Read the model definition and answer for the solid it produces. Units are mm, in the model's axes. A direction names the side the tool comes from. Give positions to 0.01 mm unless a question says otherwise; leave off trailing zeros. Loops run counter-clockwise (first coordinate to the right, second up) from the corner with the lowest first, then second, coordinate; pieces in that order, holes last.
(1) Find section C-C, the plane y = -9. Write down the section's boundary in (x, z), then the cut area to 3 significant figures.
(2) Each of these flat-tipped pins is pushed along its axis until it touches: P1, Ø6, axis at y = -26, z = 9, coming from the +X side; P2, Ø5, axis at x = 20.5, z = 4.5, coming from the -Y side. Where does it stop, or does it pass through?
(3) Find section B-B, the plane x = 18.25. Write down the section's boundary in (y, z), then the cut area to 3 significant figures.
(4) Find section D-D, the plane x = 0. Write down the section's boundary in (y, z).
(5) Find section A-A, the plane y = -31. Write down the section's boundary in (x, z), then the cut area to 3 significant figures.
(6) Determine the mould class of faces 4 (the face through (-0.521, -27.034, 5.07)), 5 (the face through (0, 40.074, 5)), 6 (the face through (-13.861, -31, 5)) for opening direction Y: pulls with the +Y half, pulls with the -Y half, needs draft (parallel to the pull), parting line crosses it, or undercut.
(7) Which of the six approach directions +Z, -Z, +X, -X, +Y, -Y give full straight-line access (tool end or side, diameter ignored) to faces 1 (the face through (0, 1, 0)), 2 (the face through (25, -21.926, 5)), 3 (the face through (-24, -21.926, 5))?
(8) Straight lines are drawn through the part: probe 1 along Y at (x, z) = (0, 5.5); probe 2 along Y at (x, z) = (-18, 7); probe 3 along X at (y, z) = (-9.5, 2). For each, find the intervals that lie inside material, in ascending order.
```python
from build123d import *

# Parameters (mm, degrees)
BOSS_EXTRUDE1_DEPTH = 10
SKETCH2_R           = 4
SKETCH2_R_2         = 2.5
CUT_EXTRUDE1_DEPTH  = 11
SKETCH8_R           = 12.955
CUT_EXTRUDE9_DEPTH  = 10


with BuildPart() as part:
    # Sketch1 → Boss-Extrude1 (new body)
    with BuildSketch(Plane.XY):
        Polygon((-35, 40.07390675), (35, 40.07390675), (35, -21.92609325), (13.861088822, -21.92609325), (13.861088822, -40.07390675), (-13.861088822, -40.07390675), (-13.861088822, -21.92609325), (-35, -21.92609325), align=None)
    extrude(amount=BOSS_EXTRUDE1_DEPTH)

    # Sketch2 → Cut-Extrude1 (cut, through all)
    with BuildSketch(Plane.XY.offset(10)):
        with Locations((0, -31)):
            Circle(SKETCH2_R)
        with Locations((0, -9)):
            Circle(SKETCH2_R)
        with Locations((-18.25, -9)):
            Circle(SKETCH2_R_2)
        with Locations((18.25, -9)):
            Circle(SKETCH2_R_2)
    extrude(amount=-CUT_EXTRUDE1_DEPTH, mode=Mode.SUBTRACT)

    # Sketch8 → Cut-Extrude9 (cut)
    with BuildSketch(Plane.XY.offset(10)):
        with Locations((0, 21.51390675)):
            Circle(SKETCH8_R)
    extrude(amount=-CUT_EXTRUDE9_DEPTH, mode=Mode.SUBTRACT)


solid = part.part
```
Entries:
1. outline: (-35, 0) - (-20.75, 0) - (-20.75, 10) - (-35, 10) - close; (-15.75, 0) - (-4, 0) - (-4, 10) - (-15.75, 10) - close; (4, 0) - (15.75, 0) - (15.75, 10) - (4, 10) - close; (20.75, 0) - (35, 0) - (35, 10) - (20.75, 10) - close
1. area: 520 mm2
2. P1: stops at x = 13.86
2. P2: stops at y = -21.93
3. outline: (-21.93, 0) - (-11.5, 0) - (-11.5, 10) - (-21.93, 10) - close; (-6.5, 0) - (40.07, 0) - (40.07, 10) - (-6.5, 10) - close
3. area: 570 mm2
4. outline: (-40.07, 0) - (-35, 0) - (-35, 10) - (-40.07, 10) - close; (-27, 0) - (-13, 0) - (-13, 10) - (-27, 10) - close; (-5, 0) - (8.56, 0) - (8.56, 10) - (-5, 10) - close; (34.47, 0) - (40.07, 0) - (40.07, 10) - (34.47, 10) - close
5. outline: (-13.86, 0) - (-4, 0) - (-4, 10) - (-13.86, 10) - close; (4, 0) - (13.86, 0) - (13.86, 10) - (4, 10) - close
5. area: 197 mm2
6. face 4: undercut
6. face 5: pulls with the +Y half
6. face 6: needs draft
7. face 1: -Z, +X, -X, +Y, -Y
7. face 2: +Z, -Z, +X, -Y
7. face 3: +Z, -Z, -X, -Y
8. probe 1: y = -40.07 to -35, -27 to -13, -5 to 8.56, 34.47 to 40.07
8. probe 2: y = -21.93 to -11.49, -6.51 to 40.07
8. probe 3: x = -35 to -20.7, -15.8 to -3.97, 3.97 to 15.8, 20.7 to 35
